CAD build for the part. Positions are in the model's coordinates, mm. Face numbers are marked on the shaded views. Coordinates: 2 decimals unless noted, no trailing zeros. Loops run counter-clockwise (first coordinate to the right, second up) from the corner with the lowest first, then second, coordinate; pieces in that order, holes last. Notation, with made-up numbers: (-15.75, 84.25) -> (-8.75, 84.25) arc R15 ccw to (-8.75, 100.25) -> close; hole circle Ø10 at (61.25, 45). An arc over 180 degrees is marked (long way). Answer as CSV lines item,"result". Start each with the question number.
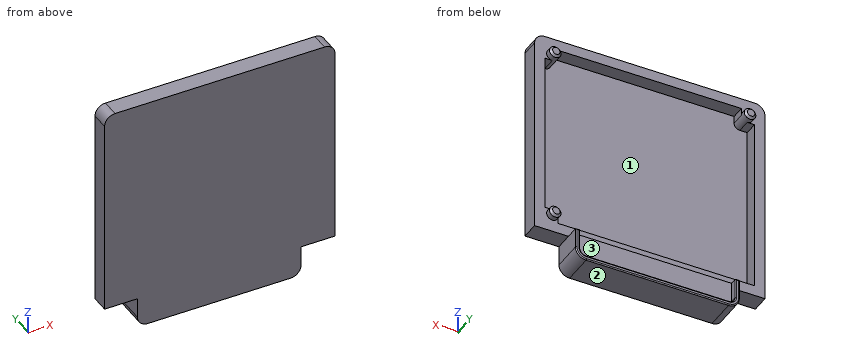
```python
from build123d import *

# Parameters (mm, degrees)
SKETCH1_W           = 110
SKETCH1_H           = 100
BOSS_EXTRUDE1_DEPTH = 2
SKETCH2_W           = 110
SKETCH2_H           = 100
SKETCH2_W_2         = 100
SKETCH2_H_2         = 90
BOSS_EXTRUDE2_DEPTH = 6.5
BOSS_EXTRUDE3_DEPTH = 13.5
BOSS_EXTRUDE4_START = -15.1
BOSS_EXTRUDE4_DEPTH = 1.6
SKETCH4_R           = 2.75
BOSS_EXTRUDE5_DEPTH = 6.5
SKETCH4_3_R         = 2.75
BOSS_EXTRUDE6_DEPTH = 10
CHAMFER1_SIZE       = 1
FILLET1_R           = 5
FILLET2_R           = 0.5
CUT_EXTRUDE1_DEPTH  = 2


# Read off the part's stored shape, not the designer's step: Boss-Extrude4
with BuildPart() as part:
    # Sketch1 → Boss-Extrude1 (new body)
    with BuildSketch(Plane(origin=(0, 0, 0), x_dir=(1, 0, 0), z_dir=(0, 1, 0))):
        Rectangle(SKETCH1_W, SKETCH1_H)
    extrude(amount=BOSS_EXTRUDE1_DEPTH)

    # Sketch2 → Boss-Extrude2 (add)
    with BuildSketch(Plane(origin=(0, 2, 0), x_dir=(1, 0, 0), z_dir=(0, 1, 0))):
        Rectangle(SKETCH2_W, SKETCH2_H)
        Rectangle(SKETCH2_W_2, SKETCH2_H_2, mode=Mode.SUBTRACT)
    extrude(amount=BOSS_EXTRUDE2_DEPTH)

    # Sketch3 → Boss-Extrude3 (add)
    with BuildSketch(Plane.XZ):
        with BuildLine():
            Line((-39.37766222, -50), (-39.37766222, -59.477632813))
            ThreePointArc((-39.37766222, -59.477632813), (-37.883906804, -63.083877397), (-34.27766222, -64.577632813))
            Line((-34.27766222, -64.577632813), (33.72233778, -64.577632813))
            ThreePointArc((33.72233778, -64.577632813), (37.328582364, -63.083877397), (38.82233778, -59.477632813))
            Line((38.82233778, -59.477632813), (38.82233778, -50))
            Line((38.82233778, -50), (-39.37766222, -50))
        make_face()
    extrude(amount=-BOSS_EXTRUDE3_DEPTH)

    # Boss-Extrude4 outline → Boss-Extrude4 (add)
    with BuildSketch(Plane.XZ.offset(BOSS_EXTRUDE4_START)):
        with BuildLine():
            Line((38.82233778, -59.477632813), (38.82233778, -50))
            Line((38.82233778, -50), (36.82233778, -50))
            Line((36.82233778, -50), (36.82233778, -59.477632813))
            ThreePointArc((36.82233778, -59.477632813), (35.914368802, -61.669663835), (33.72233778, -62.577632813))
            Line((33.72233778, -62.577632813), (-34.27766222, -62.577632813))
            ThreePointArc((-34.27766222, -62.577632813), (-36.469693242, -61.669663835), (-37.37766222, -59.477632813))
            Line((-37.37766222, -59.477632813), (-37.37766222, -50))
            Line((-37.37766222, -50), (-39.37766222, -50))
            Line((-39.37766222, -50), (-39.37766222, -59.477632813))
            ThreePointArc((-39.37766222, -59.477632813), (-37.883906804, -63.083877397), (-34.27766222, -64.577632813))
            Line((-34.27766222, -64.577632813), (33.72233778, -64.577632813))
            ThreePointArc((33.72233778, -64.577632813), (37.328582364, -63.083877397), (38.82233778, -59.477632813))
        make_face()
    extrude(amount=BOSS_EXTRUDE4_DEPTH)

    # Sketch4 → Boss-Extrude5 (add)
    with BuildSketch(Plane(origin=(0, 2, 0), x_dir=(1, 0, 0), z_dir=(0, 1, 0))):
        with BuildLine():
            Line((-50, -38.75), (-50, -45))
            Line((-50, -45), (-43.75, -45))
            Line((-43.75, -45), (-43.75, -41.5))
            ThreePointArc((-43.75, -41.5), (-48.444543648, -43.444543648), (-46.5, -38.75))
            Line((-46.5, -38.75), (-50, -38.75))
        make_face()
        with Locations((-46.5, -41.5)):
            Circle(SKETCH4_R)
        with BuildLine():
            Line((43.75, -41.5), (43.75, -45))
            Line((43.75, -45), (50, -45))
            Line((50, -45), (50, -38.75))
            Line((50, -38.75), (46.5, -38.75))
            ThreePointArc((46.5, -38.75), (48.444543648, -39.555456352), (49.25, -41.5))
            ThreePointArc((49.25, -41.5), (46.5, -44.25), (43.75, -41.5))
        make_face()
        with Locations((46.5, -41.5)):
            Circle(SKETCH4_R)
        with Locations((46.5, 41.5)):
            Circle(SKETCH4_R)
        with BuildLine():
            Line((50, 45), (43.75, 45))
            Line((43.75, 45), (43.75, 41.5))
            ThreePointArc((43.75, 41.5), (46.5, 44.25), (49.25, 41.5))
            ThreePointArc((49.25, 41.5), (48.444543648, 39.555456352), (46.5, 38.75))
            Line((46.5, 38.75), (50, 38.75))
            Line((50, 38.75), (50, 45))
        make_face()
    extrude(amount=BOSS_EXTRUDE5_DEPTH)

    # Sketch4<3> → Boss-Extrude6 (add)
    with BuildSketch(Plane(origin=(0, 2, 0), x_dir=(1, 0, 0), z_dir=(0, 1, 0))):
        with Locations(Location((46.5, 41.5, 0), (0, 0, 270))):
            Circle(SKETCH4_3_R)
        with Locations(Location((46.5, -41.5, 0), (0, 0, 90))):
            Circle(SKETCH4_3_R)
        with Locations(Location((-46.5, -41.5, 0), (0, 0, 90))):
            Circle(SKETCH4_3_R)
    extrude(amount=BOSS_EXTRUDE6_DEPTH)

    # Chamfer1
    chamfer1_edges = [part.edges().sort_by_distance(p)[0] for p in [
        (46.5, 12, -44.25),
        (46.5, 12, 44.25),
        (-46.5, 12, 44.25),
    ]]
    chamfer(chamfer1_edges, length=CHAMFER1_SIZE)

    # Fillet1
    fillet1_edges = [part.edges().sort_by_distance(p)[0] for p in [
        (55, 4.25, 50),
        (-55, 4.25, 50),
    ]]
    fillet(fillet1_edges, radius=FILLET1_R)

    # Fillet2
    fillet2_edges = [part.edges().sort_by_distance(p)[0] for p in [
        (35.914368802, 15.1, -61.669663835),
        (37.82233778, 15.1, -50),
        (38.82233778, 15.1, -54.738816406),
        (-0.27766222, 15.1, -64.577632813),
        (-39.37766222, 15.1, -54.738816406),
        (-38.37766222, 15.1, -50),
        (-36.469693242, 15.1, -61.669663835),
        (-0.27766222, 15.1, -62.577632813),
        (-37.37766222, 15.1, -54.738816406),
        (-37.883906804, 15.1, -63.083877397),
        (37.328582364, 15.1, -63.083877397),
        (36.82233778, 15.1, -54.738816406),
    ]]
    fillet(fillet2_edges, radius=FILLET2_R)

    # Sketch5 → Cut-Extrude1 (cut)
    with BuildSketch(Plane(origin=(0, 13.5, 0), x_dir=(1, 0, 0), z_dir=(0, 1, 0))):
        with BuildLine():
            Line((-37.37766222, 59.477632813), (-37.37766222, 50))
            Line((-37.37766222, 50), (36.82233778, 50))
            Line((36.82233778, 50), (36.82233778, 59.477632813))
            ThreePointArc((36.82233778, 59.477632813), (35.914368802, 61.669663835), (33.72233778, 62.577632813))
            Line((33.72233778, 62.577632813), (-34.27766222, 62.577632813))
            ThreePointArc((-34.27766222, 62.577632813), (-36.469693242, 61.669663835), (-37.37766222, 59.477632813))
        make_face()
    extrude(amount=-CUT_EXTRUDE1_DEPTH, mode=Mode.SUBTRACT)


solid = part.part
```
Q1. Saw through at A-A (y = 4). List the corners of the cut face in (x, z).
Q2. Saw through at C-C (z = 21.5). List the corners of the cut face in (x, y), and give its area (3 significant figures).
Q3. Probe probe 1 along Z at (x, y) = (-3, 7.75); probe 2 along X at (y, z) = (3.5, -28.5); probe 3 along X at (y, z) = (7, 44.5). List the from-to ranges inside material, lowest first. Write a range as from..to.
Q4. Pin check, flat tips, straight feed: pin 1 Ø5 at (x, y) = (-4.5, 11.5) entering from +Z; pin 2 Ø12 at (x, z) = (-23.5, -9) entering from +Y; pin 3 Ø1 at (x, z) = (-46, 42) entering from +Y. Stop position of each tip, or through.
Q5. Saw through at B-B (x = 0.5). List the corners of the cut face in (y, z), and give its area (3 significant figures).
Q6. Two-plate mould, pull along Z, no slides. Class the marked faces 1, 2 and 3: pulls with the +Z half, pulls with the -Z half, needs draft (parallel to the pull), parting line crosses it, or undercut.
Ans:
1,outline,"(-55, -50) -> (-39.38, -50) -> (-39.38, -59.48) arc R5.1 ccw to (-34.28, -64.58) -> (33.72, -64.58) arc R5.1 ccw to (38.82, -59.48) -> (38.82, -50) -> (55, -50) -> (55, 45) arc R5 ccw to (50, 50) -> (-50, 50) arc R5 ccw to (-55, 45) -> close; hole (-50, -45) -> (43.75, -45) -> (43.75, -41.5) arc R2.75 cw to (46.5, -38.75) -> (50, -38.75) -> (50, 38.75) -> (46.5, 38.75) arc R2.75 cw to (43.75, 41.5) -> (43.75, 45) -> (-43.75, 45) -> (-43.75, 41.5) arc R2.75 cw to (-46.5, 38.75) -> (-50, 38.75) -> close"
2,outline,"(-55, 0) -> (55, 0) -> (55, 8.5) -> (50, 8.5) -> (50, 2) -> (-50, 2) -> (-50, 8.5) -> (-55, 8.5) -> close"
2,area,"285 mm²"
3,probe 1,"z = -64.58..-45, 45..50"
3,probe 2,"x = -55..-50, 50..55"
3,probe 3,"x = -55..-43.75, 43.75..55"
4,pin 1,"stops at z = -50"
4,pin 2,"stops at y = 2"
4,pin 3,"stops at y = 12"
5,outline,"(0, -64.58) -> (14.6, -64.58) arc R0.5 ccw to (15.1, -64.08) -> (15.1, -63.08) arc R0.5 ccw to (14.6, -62.58) -> (11.5, -62.58) -> (11.5, -50) -> (8.5, -50) -> (8.5, -45) -> (2, -45) -> (2, 45) -> (8.5, 45) -> (8.5, 50) -> (0, 50) -> close"
5,area,"440 mm²"
6,face 1,"undercut"
6,face 2,"pulls with the -Z half"
6,face 3,"needs draft"
